```python
from build123d import *

# Parameters (mm, degrees)
F1_DEPTH  = 150
F2_R      = 20.6152991637
F3_DEPTH  = 30
F3_FACE_R = 20.6152991637
F4_DEPTH  = 25
F4_TAPER  = -45


with BuildPart() as f1:
    # F0 (on Front) → F1 (new body)
    with BuildSketch(Plane.XZ):
        Polygon((4.725022344, -22.3287471763), (19.1299038845, -12.447713203), (22.3287471763, 4.725022344), (12.447713203, 19.1299038845), (-4.725022344, 22.3287471763), (-19.1299038845, 12.447713203), (-22.3287471763, -4.725022344), (-12.447713203, -19.1299038845), align=None)
    extrude(amount=F1_DEPTH)

    # F2 (on face) → F3 (join)
    with BuildSketch(Plane(origin=(0, 0, 0), x_dir=(-1, 0, 0), z_dir=(0, 1, 0))):
        Circle(F2_R)
    extrude(amount=F3_DEPTH)

    # F3_face (on face) → F4 (join)
    with BuildSketch(Plane(origin=(0, 30, 0), x_dir=(-1, 0, 0), z_dir=(0, 1, 0))):
        Circle(F3_FACE_R)
    extrude(amount=F4_DEPTH, taper=F4_TAPER)


solid = f1.part
```
Here's how the part is built. I have some questions about the finished solid (model axes, mm). A direction names the side the tool comes from. Round coordinates to 2 decimals unless told otherwise and drop trailing zeros. Loops run counter-clockwise (first coordinate to the right, second up) from the corner with the lowest first, then second, coordinate; pieces in that order, holes last.
1. Thinking about a two-plate mould opening in Y: for faces 1 (the face through (4.469, 14.79, -20.125)), 2 (the face through (0, -150, 0)), 3 (the face through (-11.827, -73.95, 17.457)), 4 (the face through (7, 0, -20)), which applies, released by +Y, released by -Y, zero draft, split by the parting line, or undercut?
Answers:
face 1: undercut
face 2: released by -Y
face 3: zero draft
face 4: undercut
2. Suppose I cut it at A-A, the plane y = -52.5. Please give me the cut outline in (x, z).
Answers:
outline: (-22.33, -4.73) - (-12.45, -19.13) - (4.73, -22.33) - (19.13, -12.45) - (22.33, 4.73) - (12.45, 19.13) - (-4.73, 22.33) - (-19.13, 12.45) - close
3. For faces 5 (the face through (-17.457, -73.95, -11.827)), 6 (the face through (-20.707, -73.95, 3.982)), 7 (the face through (3.982, -73.95, 20.707)), 8 (the face through (20.707, -73.95, -3.982)), which set-ups out of +Z, -Z, +X, -X, +Y, -Y let a thin tool reach every point of the face, with its end or its side?
Answers:
face 5: -Z, -X, -Y
face 6: +Z, -X, -Y
face 7: +Z, +X, -Y
face 8: -Z, +X, -Y
4. Suppose I cut it at B-B, the plane x = 0. Please give me the cut outline in (y, z).
Answers:
outline: (-150, -21.45) - (0, -21.45) - (0, -20.62) - (30, -20.62) - (55, -45.62) - (55, 45.62) - (30, 20.62) - (0, 20.62) - (0, 21.45) - (-150, 21.45) - close
5. Suppose I cut it at C-C, the plane y = 38. Please give me the cut outline in (x, z), and give its area (3 significant figures).
Answers:
outline: circle Ø57.23 at (0, 0)
area: 2,570 mm2
6. If I drill on probe 1 along X at (y, z) = (-65, 4.5); probe 2 along Y at (x, z) = (11, 17.5); probe 3 along X at (y, z) = (-109, 2.5), over which ranges is the centre line in solid material (lowest first)?
Answers:
probe 1: x = -20.61 to 22.29
probe 2: y = -150 to 0, 30.05 to 55
probe 3: x = -20.98 to 21.91
7. Will these pins go through, and if not, where does the flat tip stop? pin 1 (8 mm diameter, centred on x = -17, y = -28, fed in from +Z); pin 2 (3 mm diameter, centred on x = -15.5, y = -3.5, fed in from +Z); pin 3 (1 mm diameter, centred on y = -69.5, z = -6.5, fed in from -X).
Answers:
pin 1: stops at z = 16.65
pin 2: stops at z = 15.97
pin 3: stops at x = -21.45
